The model under review builds one solid part; all positions refer to its coordinate system, in mm. Give positions to 0.01 mm unless a question says otherwise; leave off trailing zeros. Write each loop counter-clockwise with the first axis right and the second up, starting at its lowest first coordinate (ties: lowest second). Pieces come first, ordered by that corner, then holes. Notation, with made-up numbers: (2, 24) - (7, 24) arc R19 cw to (7, 31) - close; hole circle Ø10 at (23, 68). An arc over 180 degrees is marked (long way). Write item = value, one per line.
```python
from build123d import *

# Parameters (mm, degrees)
BOSS_EXTRUDE1_DEPTH = 10
SKETCH2_R           = 6.5
SKETCH2_R_2         = 5
CUT_EXTRUDE1_DEPTH  = 6.5
BOSS_EXTRUDE2_DEPTH = 3.5
SKETCH4_W           = 1.5
SKETCH4_H           = 75.5
CUT_EXTRUDE2_DEPTH  = 11


with BuildPart() as part:
    # Sketch1 → Boss-Extrude1 (new body)
    with BuildSketch(Plane.XY):
        with BuildLine():
            Line((-50, -86), (50, -86))
            Line((50, -86), (5, 0))
            Line((5, 0), (2.5, 0))
            ThreePointArc((2.5, 0), (0, -2.5), (-2.5, 0))
            Line((-2.5, 0), (-5, 0))
            Line((-5, 0), (-50, -86))
        make_face()
    extrude(amount=BOSS_EXTRUDE1_DEPTH)

    # Sketch2 → Cut-Extrude1 (cut)
    with BuildSketch(Plane.XY.offset(10)):
        Circle(SKETCH2_R)
        Circle(SKETCH2_R_2, mode=Mode.SUBTRACT)
    extrude(amount=-CUT_EXTRUDE1_DEPTH, mode=Mode.SUBTRACT)

    # Sketch3 → Boss-Extrude2 (add)
    with BuildSketch(Plane.XY.offset(10)):
        with BuildLine():
            Line((5, 0), (6.130459134, -2.160433012))
            ThreePointArc((6.130459134, -2.160433012), (0, -6.5), (-6.130459134, -2.160433012))
            Line((-6.130459134, -2.160433012), (-5, 0))
            ThreePointArc((-5, 0), (0, -5), (5, 0))
        make_face()
    extrude(amount=-BOSS_EXTRUDE2_DEPTH)

    # Sketch4 → Cut-Extrude2 (cut, through all)
    with BuildSketch(Plane.XY.offset(10)):
        with Locations((0, -46.25)):
            Rectangle(SKETCH4_W, SKETCH4_H)
    extrude(amount=-CUT_EXTRUDE2_DEPTH, mode=Mode.SUBTRACT)


solid = part.part
```
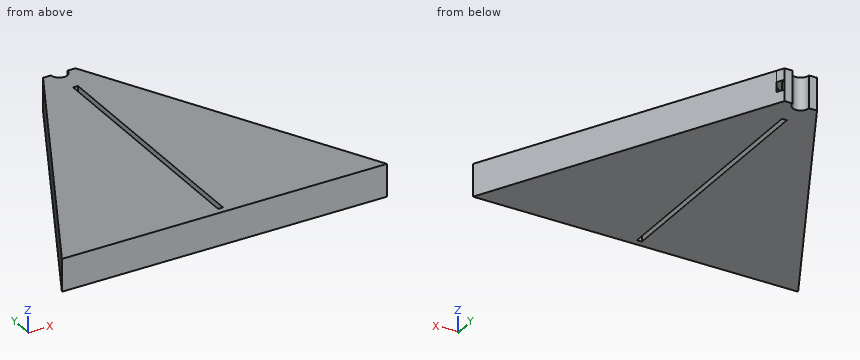
1. For line 1 (X direction, y = -11.5, z = 6.25); line 2 (X direction, y = -75, z = 1.25); line 3 (Y direction, x = -35.5, z = 6.25), list the stretches that pass through material, from the lowest coordinate up. Write a range as from..to.
Findings below:
line_1 = -11.02..-0.75, 0.75..11.02
line_2 = -44.24..-0.75, 0.75..44.24
line_3 = -86..-58.29
2. Take a section at D-D on x = 29. Give the boundary of the cut face in (y, z).
Findings below:
outline = (-86, 0) - (-45.87, 0) - (-45.87, 10) - (-86, 10) - close
3. Insertion check: P1, Ø3, axis at x = -36, z = 4.5, coming from the +Y side; P2, Ø1.2, axis at x = -0.5, z = 4.5, coming from the +Y side (3 decimals); P3, Ø6, axis at y = -61, z = 1.5, coming from the -X side. Each pin has a flat end and moves straight along its axis. Give the tip position at first contact, or say it passes through.
Findings below:
P1 = -56.38
P2 = -2.245
P3 = -38.49
4. Take a section at C-C on y = -32.5. Give the boundary of the cut face in (x, z).
Findings below:
outline = (-22.01, 0) - (-0.75, 0) - (-0.75, 10) - (-22.01, 10) - close; (0.75, 0) - (22.01, 0) - (22.01, 10) - (0.75, 10) - close
5. Take a section at A-A on y = -64.5. Give the boundary of the cut face in (x, z), and give its area (3 significant figures).
Findings below:
outline = (-38.75, 0) - (-0.75, 0) - (-0.75, 10) - (-38.75, 10) - close; (0.75, 0) - (38.75, 0) - (38.75, 10) - (0.75, 10) - close
area = 760 mm²
6. Take a section at B-B on z = 7.75. Give the boundary of the cut face in (x, y), and give its area (3 significant figures).
Findings below:
outline = (-50, -86) - (50, -86) - (5, 0) - (2.5, 0) arc R2.5 cw to (-2.5, 0) - (-5, 0) - close; hole (-0.75, -84) - (0.75, -84) - (0.75, -8.5) - (-0.75, -8.5) - close
area = 4,610 mm²
